Read the model definition and answer for the solid it produces. Units are mm, in the model's axes. A direction names the side the tool comes from. Coordinates: 2 decimals unless noted, no trailing zeros. Write each loop counter-clockwise with the first axis right and the second up, starting at its lowest first coordinate (ties: lowest second). Pieces come first, ordered by that corner, then holes. Notation, with made-up numbers: M 66,-37.5 L 105,-37.5 A9 cw 105,-25.5 Z; hole C 3.5,44.5 d2. An arc over 180 degrees is marked long. Write item = value, one per line.
from build123d import *

# Parameters (mm, degrees)
SKETCH1_W           = 45
SKETCH1_H           = 26
BOSS_EXTRUDE1_DEPTH = 5
SKETCH2_W           = 2.5
SKETCH2_H           = 26
BOSS_EXTRUDE2_DEPTH = 70
LPATTERN2_COUNT     = 2
LPATTERN2_PITCH     = 42.5
SKETCH3_W           = 45
SKETCH3_H           = 26
BOSS_EXTRUDE3_DEPTH = 5
SKETCH7_R           = 10.5
BOSS_EXTRUDE5_DEPTH = 10
LPATTERN3_COUNT     = 2
LPATTERN3_PITCH     = 50
CUT_EXTRUDE1_REACH  = 105.325
SKETCH8_R           = 1.2
CIRPATTERN1_COUNT   = 4
SKETCH9_R           = 3
CUT_EXTRUDE2_DEPTH  = 2
BOSS_EXTRUDE6_START = 5
SKETCH10_R          = 10.5
BOSS_EXTRUDE6_DEPTH = 5
SKETCH11_W          = 40
SKETCH11_H          = 5
BOSS_EXTRUDE7_DEPTH = 50
FILLET1_R           = 10
SKETCH12_R          = 3
SKETCH12_R_2        = 1.2
CUT_EXTRUDE3_DEPTH  = 50
CIRPATTERN2_COUNT   = 4


with BuildPart() as part:
    # Sketch1 → Boss-Extrude1 (new body)
    with BuildSketch(Plane(origin=(0, 0, 0), x_dir=(1, 0, 0), z_dir=(0, 1, 0))):
        with Locations((22.5, 13)):
            Rectangle(SKETCH1_W, SKETCH1_H)
    extrude(amount=BOSS_EXTRUDE1_DEPTH)

    # Sketch2 → Boss-Extrude2 (add)
    with BuildSketch(Plane(origin=(0, 5, 0), x_dir=(1, 0, 0), z_dir=(0, 1, 0))):
        with Locations((1.25, 13)):
            Rectangle(SKETCH2_W, SKETCH2_H)
    boss_extrude2 = extrude(amount=BOSS_EXTRUDE2_DEPTH)

    # LPattern2: Boss-Extrude2 ×2
    with Locations(*[(i * LPATTERN2_PITCH, 0, 0) for i in range(1, LPATTERN2_COUNT)]):
        add(boss_extrude2)

    # Sketch3 → Boss-Extrude3 (add)
    with BuildSketch(Plane(origin=(0, 75, 0), x_dir=(1, 0, 0), z_dir=(0, 1, 0))):
        with Locations((22.5, 13)):
            Rectangle(SKETCH3_W, SKETCH3_H)
    extrude(amount=BOSS_EXTRUDE3_DEPTH)

    # Sketch7 → Boss-Extrude5 (add)
    with BuildSketch(Plane.ZY):
        with Locations((-13, 40)):
            Circle(SKETCH7_R)
    boss_extrude5 = extrude(amount=BOSS_EXTRUDE5_DEPTH)

    # LPattern3: Boss-Extrude5 ×2
    with Locations(*[(i * LPATTERN3_PITCH, 0, 0) for i in range(1, LPATTERN3_COUNT)]):
        add(boss_extrude5)

    # Sketch8 → Cut-Extrude1 (cut, up to next)
    with BuildSketch(Plane.ZY.offset(10), mode=Mode.PRIVATE) as cut_extrude1_sk1:
        with Locations((-13, 47)):
            Circle(SKETCH8_R)
    cut_extrude1_tool1 = extrude(cut_extrude1_sk1.sketch, amount=-CUT_EXTRUDE1_REACH, mode=Mode.PRIVATE) & part.part
    cut_extrude1 = cut_extrude1_tool1.solids().sort_by_distance((-10, 47, -13))[0]
    add(cut_extrude1, mode=Mode.SUBTRACT)

    # CirPattern1: Cut-Extrude1 ×4 about axis
    cirpattern1_axis = Axis((0, 40, -13), (1, 0, 0))
    for i in range(1, CIRPATTERN1_COUNT):
        add(cut_extrude1.rotate(cirpattern1_axis, i * 360 / CIRPATTERN1_COUNT), mode=Mode.SUBTRACT)

    # Sketch9 → Cut-Extrude2 (cut)
    with BuildSketch(Plane.ZY.offset(10)):
        with Locations((-13, 40)):
            Circle(SKETCH9_R)
    extrude(amount=-CUT_EXTRUDE2_DEPTH, mode=Mode.SUBTRACT)

    # Sketch10 → Boss-Extrude6 (add)
    with BuildSketch(Plane(origin=(50, 0, 0), x_dir=(0, 0, -1), z_dir=(1, 0, 0)).offset(BOSS_EXTRUDE6_START)):
        with Locations(Location((13, 40, 0), (0, 0, 180))):
            Circle(SKETCH10_R)
    extrude(amount=-BOSS_EXTRUDE6_DEPTH)

    # Sketch11 → Boss-Extrude7 (add)
    with BuildSketch(Plane(origin=(0, 0, -26), x_dir=(-1, 0, 0), z_dir=(0, 0, -1))):
        with Locations((-22.5, 77.5)):
            Rectangle(SKETCH11_W, SKETCH11_H)
    extrude(amount=BOSS_EXTRUDE7_DEPTH)

    # Fillet1
    # the kernel refuses this fillet: 10 mm, written as the material it adds along each edge
    with BuildSketch(Plane(origin=(2.5, 80, -26), x_dir=(-1, 0, 0), z_dir=(0, -1, 0)), Plane(origin=(42.5, 75, -26), x_dir=(1, 0, 0), z_dir=(0, 1, 0))) as fillet1_piece_1:
        with BuildLine():
            CenterArc((10, 6.614378278), FILLET1_R, 180, 41.409622109)
            Line((0, 6.614378278), (0, 0))
            Line((0, 0), (2.5, 0))
        make_face()
    extrude(amount=5)
    # the kernel refuses this fillet: 10 mm, written as the material it takes off along each edge
    with BuildSketch(Plane(origin=(2.5, 105, -76), x_dir=(0, 0, 1), z_dir=(0, -1, 0))) as fillet1_2_piece_1:
        with BuildLine():
            CenterArc((FILLET1_R, -FILLET1_R), FILLET1_R, 90, 90)
            Line((0, -FILLET1_R), (0, 0))
            Line((0, 0), (FILLET1_R, 0))
        make_face()
    extrude(amount=55, mode=Mode.SUBTRACT)
    with BuildSketch(Plane(origin=(42.5, 50, -76), x_dir=(-1, 0, 0), z_dir=(0, 1, 0))) as fillet1_2_piece_2:
        with BuildLine():
            CenterArc((FILLET1_R, FILLET1_R), FILLET1_R, 180, 90)
            Line((0, FILLET1_R), (0, 0))
            Line((0, 0), (FILLET1_R, 0))
        make_face()
    extrude(amount=55, mode=Mode.SUBTRACT)

    # Sketch12 → Cut-Extrude3 (cut)
    with BuildSketch(Plane(origin=(0, 80, 0), x_dir=(1, 0, 0), z_dir=(0, 1, 0))):
        with Locations(Location((22.5, 60, 0), (0, 0, 270))):
            Circle(SKETCH12_R)
        with Locations(Location((29.5, 60, 0), (0, 0, 270))):
            Circle(SKETCH12_R_2)
    cut_extrude3 = extrude(amount=-CUT_EXTRUDE3_DEPTH, mode=Mode.SUBTRACT)

    # CirPattern2: Cut-Extrude3 ×4 about axis
    cirpattern2_axis = Axis((22.5, 0, -60), (0, 1, 0))
    for i in range(1, CIRPATTERN2_COUNT):
        add(cut_extrude3.rotate(cirpattern2_axis, i * 360 / CIRPATTERN2_COUNT), mode=Mode.SUBTRACT)


solid = part.part
Item 1: For a pull along Z with two mould halves and no side action, classify faces 4 (the face through (22, 5, -13)), 5 (the face through (23, 78, -76)), 6 (the face through (-3.84, 48.19, -13.16)) as released by +Z, released by -Z, zero draft, split by the parting line, or undercut.
Worked answers:
face_4 = zero draft
face_5 = released by -Z
face_6 = undercut
Item 2: Find section C-C (y = 40). State how many separate pieces and enclosed holes the cut face has, and give its area (4 significant figures).
Worked answers:
separate_pieces = 4
enclosed_holes = 0
area = 530.5 mm²
Item 3: Find section D-D (x = 29.5). Determine the outline of the cut face in (y, z).
Worked answers:
outline = M 0,-26 L 5,-26 L 5,0 L 0,0 Z; M 75,-76 L 80,-76 L 80,-61.2 L 75,-61.2 Z; M 75,-58.8 L 80,-58.8 L 80,0 L 75,0 Z
Item 4: Consider line 1 along X through (y, z) = (78, -60); line 2 along Z through (x, y) = (22.5, 78.25); line 3 along X through (y, z) = (55.5, -7). Determine where each line is inside the solid, lowest interval first. Write a range as from..to.
Worked answers:
line_1 = 2.5..14.3, 16.7..19.5, 25.5..28.3, 30.7..42.5
line_2 = -76..-68.2, -65.8..-63, -57..-54.2, -51.8..0
line_3 = 0..2.5, 42.5..45
Item 5: Find section A-A (x = 22.5). Determine the outline of the cut face in (y, z), and give its area (3 significant figures).
Worked answers:
outline = M 0,-26 L 5,-26 L 5,0 L 0,0 Z; M 75,-76 L 80,-76 L 80,-68.2 L 75,-68.2 Z; M 75,-65.8 L 80,-65.8 L 80,-63 L 75,-63 Z; M 75,-57 L 80,-57 L 80,-54.2 L 75,-54.2 Z; M 75,-51.8 L 80,-51.8 L 80,0 L 75,0 Z
area = 456 mm²
Item 6: Find section B-B (z = -53). Determine the outline of the cut face in (x, y).
Worked answers:
outline = M 2.5,75 L 21.3,75 L 21.3,80 L 2.5,80 Z; M 23.7,75 L 42.5,75 L 42.5,80 L 23.7,80 Z
Item 7: Which of the six approach directions +Z, -Z, +X, -X, +Y, -Y give full straight-line access (tool end or side, diameter ignored) to faces 1 (the face through (-4.93, 30.685, -8.155)), 2 (the face through (2.5, 77, -49)), 3 (the face through (40, 40, -13))?
Worked answers:
face_1 = -X
face_2 = -Z, -X, +Y, -Y
face_3 = +Z, -Z
Item 8: Flat-ended cylindrical pins translate along their axes: pin 1 (22.5 mm diameter, centred on x = 27, y = 51, fed in from -Z); pin 2 (13 mm diameter, centred on y = 59.5, z = -13.5, fed in from -X); pin 3 (2.5 mm diameter, centred on y = 77.5, z = -52.5, fed in from -X); pin 4 (2.5 mm diameter, centred on y = 78.5, z = -45, fed in from +X). Find the tip coordinate at first contact, or state that the pin passes through.
Worked answers:
pin_1 = through
pin_2 = 0
pin_3 = 2.5
pin_4 = 42.5
